Autodesk Inventor part; units mm, degrees
ref_plane "YZ Plane" through (0, 0, 0) normal (1, 0, 0) x (0, 1, 0)
ref_plane "XZ Plane" through (0, 0, 0) normal (0, 1, 0) x (-1, 0, 0)
ref_plane "XY Plane" through (0, 0, 0) normal (0, 0, 1) x (1, 0, 0)
sketch "Sketch1" plane through (0, 0, 0) normal (1, 0, 0) x (0, 1, 0)
  line L0 (0, 0) -> (125, 0)
  line L1 (125, 0) -> (125, 65)
  line L2 (125, 65) -> (0, 65)
  line L3 (0, 65) -> (0, 0)
  line L4 (2.875, 56.9) -> (9.125, 56.9)
  line L5 (9.125, 56.9) -> (9.125, 8.1)
  line L6 (9.125, 8.1) -> (2.875, 8.1)
  line L7 (2.875, 8.1) -> (2.875, 56.9)
  circle A0 centre (112.5, 12.5) radius 2.7
  circle A1 centre (21.5, 12.5) radius 2.7
  dimension "d0" = 65
  dimension "d1" = 125
  dimension "d2" = 6.25
  dimension "d3" = 2.875
  dimension "d4" = 8.1
  dimension "d5" = 8.1
  dimension "d6" = 12.5
  dimension "d7" = 21.5
  dimension "d8" = 12.5
  dimension "d9" = 5.4
extrude "Extrusion1" add sketch "Sketch1" along normal blind 6
fillet "Fillet1" radius 2 4 edges at (3, 125, 65) (3, 125, 0) (3, 0, 65) (3, 0, 0)
equation "\"d5\" = d4"
properties part number "FrontLeft"
CAD build for the part. Positions are in the model's coordinates, mm. A direction names the side the tool comes from. Give positions to 0.01 mm unless a question says otherwise; leave off trailing zeros. Order: outer loops, then holes, each group sorted by start corner. A loop starts at its lowest first (then second) coordinate and runs counter-clockwise, first axis right, second up. Notation, with made-up numbers: (-21, 79) -> (22, 79) arc R37 cw to (22, 115) -> close; hole circle Ø9 at (-9, 47). An arc over 180 degrees is marked (long way). Return JSON: item names as keys, results as strings.
Q1. Flat gauge pin, fed straight in: pin 1 (5 mm diameter, centred on y = 21.5, z = 12.5, fed in from +X). Where does the tip first touch, or does it go through?
Working result:
{"pin 1": "through"}
Q2. Saw through at A-A (z = 28). Write the cut outline in (x, y) (3 decimals), then the cut area to 4 significant figures.
Working result:
{"outline": "(0, 0) -> (6, 0) -> (6, 2.875) -> (0, 2.875) -> close; (0, 9.125) -> (6, 9.125) -> (6, 125) -> (0, 125) -> close", "area": "712.5 mm²"}
Q3. Mould opens along Y. For faces 3 (the face through (3, 0, 33)), 4 (the face through (3, 9.125, 33)), 5 (the face through (3, 62, 0)) say: pulls with the +Y half, pulls with the -Y half, needs draft (parallel to the pull), parting line crosses it, or undercut.
Working result:
{"face 3": "pulls with the -Y half", "face 4": "undercut", "face 5": "needs draft"}
Q4. Saw through at B-B (z = 12.5). Write the cut outline in (x, y) (3 decimals), then the cut area to 3 significant figures.
Working result:
{"outline": "(0, 0) -> (6, 0) -> (6, 2.875) -> (0, 2.875) -> close; (0, 9.125) -> (6, 9.125) -> (6, 18.8) -> (0, 18.8) -> close; (0, 24.2) -> (6, 24.2) -> (6, 109.8) -> (0, 109.8) -> close; (0, 115.2) -> (6, 115.2) -> (6, 125) -> (0, 125) -> close", "area": "648 mm²"}
Q5. Which spindle directions (+Z, -Z, +X, -X, +Y, -Y) get a long thin tool onto all of the face, cutting with end or side? Do faces 1 (the face through (6, 62, 33)), 2 (the face through (3, 2.875, 32)). Say none if no direction does.
Working result:
{"face 1": "+Z, -Z, +X, +Y, -Y", "face 2": "+X, -X"}
Q6. Saw through at C-C (y = 21.5). Write the cut outline in (x, z), then the cut area to 3 significant figures.
Working result:
{"outline": "(0, 0) -> (6, 0) -> (6, 9.8) -> (0, 9.8) -> close; (0, 15.2) -> (6, 15.2) -> (6, 65) -> (0, 65) -> close", "area": "358 mm²"}
Q7. Saw through at D-D (x = 3.6). Write the cut outline in (y, z) (3 decimals).
Working result:
{"outline": "(0, 2) arc R2 ccw to (2, 0) -> (123, 0) arc R2 ccw to (125, 2) -> (125, 63) arc R2 ccw to (123, 65) -> (2, 65) arc R2 ccw to (0, 63) -> close; hole (2.875, 8.1) -> (9.125, 8.1) -> (9.125, 56.9) -> (2.875, 56.9) -> close; hole circle Ø5.4 at (21.5, 12.5); hole circle Ø5.4 at (112.5, 12.5)"}
Q8. Drill centre lines: line 1 (Y direction, x = 5.15, z = 26) (3 decimals); line 2 (Z direction, x = 3.6, y = 21.5); line 3 (Z direction, x = 1.35, y = 20) (3 decimals). Where is each one in solid material? Low to high.
Working result:
{"line 1": "0 to 2.875, 9.125 to 125", "line 2": "0 to 9.8, 15.2 to 65", "line 3": "0 to 10.255, 14.745 to 65"}
